```python
from build123d import *

# Parameters (mm, degrees)
BOSS_EXTRUDE1_DEPTH             = 50
BOSS_EXTRUDE2_START             = -50
BOSS_EXTRUDE2_DEPTH             = 50
F_5_0MM_CLEARANCE_DOWEL_HOLE1_D = 5
CUT_EXTRUDE1_REACH              = 67.4
SKETCH4_R                       = 5
CUT_EXTRUDE2_REACH              = 68.728
CUT_EXTRUDE3_DEPTH              = 68.194679971
TAP_DRILL_FOR_M5X0_8_TAP1_D     = 4.2
TAP_DRILL_FOR_M5X0_8_TAP1_DEPTH = 8
TAP_DRILL_FOR_M5X0_8_TAP1_TIP   = 1.2618073


with BuildPart() as part:
    # Sketch1 → Boss-Extrude1 (new body)
    with BuildSketch(Plane.XY):
        with BuildLine():
            Line((-31.734248061, 1), (-17.721808598, 1))
            ThreePointArc((-17.721808598, 1), (0, 17.75), (17.721808598, 1))
            Line((17.721808598, 1), (31.734248061, 1))
            ThreePointArc((31.734248061, 1), (0, 31.75), (-31.734248061, 1))
        make_face()
    extrude(amount=BOSS_EXTRUDE1_DEPTH)

    # Sketch9 → Boss-Extrude2 (add)
    with BuildSketch(Plane.XY.offset(50).offset(BOSS_EXTRUDE2_START)):
        with BuildLine():
            Line((31.734248061, 31.75), (0, 31.75))
            ThreePointArc((0, 31.75), (22.094258304, 22.801452805), (31.734248061, 1))
            Line((31.734248061, 1), (31.734248061, 31.75))
        make_face()
        with BuildLine():
            Line((-31.734248061, 31.75), (-31.734248061, 1))
            ThreePointArc((-31.734248061, 1), (-22.094258304, 22.801452805), (0, 31.75))
            Line((0, 31.75), (-31.734248061, 31.75))
        make_face()
    extrude(amount=BOSS_EXTRUDE2_DEPTH)

    # Ø5.0mm Clearance Dowel Hole1 (through all)
    with Locations(Plane(origin=(-24.72802833, 1, 40), x_dir=(0, 0, -1), z_dir=(0, -1, 0))):
        with Locations((0, 0), (30, 0), (0, 49.45605666), (30, 49.45605666)):
            Hole(F_5_0MM_CLEARANCE_DOWEL_HOLE1_D / 2)

    # Sketch4 → Cut-Extrude1 (cut, up to next)
    with BuildSketch(Plane(origin=(0, 4, 0), x_dir=(-1, 0, 0), z_dir=(0, -1, 0)), mode=Mode.PRIVATE) as cut_extrude1_sk1:
        with Locations(Location((24.72802833, -40, 0), (0, 0, 90))):
            Circle(SKETCH4_R)
    cut_extrude1_tool1 = extrude(cut_extrude1_sk1.sketch, amount=-CUT_EXTRUDE1_REACH, mode=Mode.PRIVATE) & part.part
    # Sketch4 → Cut-Extrude1 (cut, up to next)
    with BuildSketch(Plane(origin=(0, 4, 0), x_dir=(-1, 0, 0), z_dir=(0, -1, 0)), mode=Mode.PRIVATE) as cut_extrude1_sk2:
        with Locations(Location((24.72802833, -10, 0), (0, 0, 90))):
            Circle(SKETCH4_R)
    cut_extrude1_tool2 = extrude(cut_extrude1_sk2.sketch, amount=-CUT_EXTRUDE1_REACH, mode=Mode.PRIVATE) & part.part
    # Sketch4 → Cut-Extrude1 (cut, up to next)
    with BuildSketch(Plane(origin=(0, 4, 0), x_dir=(-1, 0, 0), z_dir=(0, -1, 0)), mode=Mode.PRIVATE) as cut_extrude1_sk3:
        with Locations(Location((-24.72802833, -10, 0), (0, 0, 90))):
            Circle(SKETCH4_R)
    cut_extrude1_tool3 = extrude(cut_extrude1_sk3.sketch, amount=-CUT_EXTRUDE1_REACH, mode=Mode.PRIVATE) & part.part
    # Sketch4 → Cut-Extrude1 (cut, up to next)
    with BuildSketch(Plane(origin=(0, 4, 0), x_dir=(-1, 0, 0), z_dir=(0, -1, 0)), mode=Mode.PRIVATE) as cut_extrude1_sk4:
        with Locations(Location((-24.72802833, -40, 0), (0, 0, 90))):
            Circle(SKETCH4_R)
    cut_extrude1_tool4 = extrude(cut_extrude1_sk4.sketch, amount=-CUT_EXTRUDE1_REACH, mode=Mode.PRIVATE) & part.part
    add(cut_extrude1_tool1.solids().sort_by_distance((-24.728028, 4, 40))[0], mode=Mode.SUBTRACT)
    add(cut_extrude1_tool2.solids().sort_by_distance((-24.728028, 4, 10))[0], mode=Mode.SUBTRACT)
    add(cut_extrude1_tool3.solids().sort_by_distance((24.728028, 4, 10))[0], mode=Mode.SUBTRACT)
    add(cut_extrude1_tool4.solids().sort_by_distance((24.728028, 4, 40))[0], mode=Mode.SUBTRACT)

    # Sketch5 → Cut-Extrude2 (cut, up to next)
    with BuildSketch(Plane(origin=(0, 1, 0), x_dir=(-1, 0, 0), z_dir=(0, -1, 0)), mode=Mode.PRIVATE) as cut_extrude2_sk1:
        with BuildLine():
            Line((-6, -35), (-6, -15))
            ThreePointArc((-6, -15), (0, -9), (6, -15))
            Line((6, -15), (6, -35))
            ThreePointArc((6, -35), (0, -41), (-6, -35))
        make_face()
    cut_extrude2_tool1 = extrude(cut_extrude2_sk1.sketch, amount=-CUT_EXTRUDE2_REACH, mode=Mode.PRIVATE) & part.part
    add(cut_extrude2_tool1.solids().sort_by_distance((0, 1, 25))[0], mode=Mode.SUBTRACT)

    # Sketch6 → Cut-Extrude3 (cut, through all)
    with BuildSketch(Plane.XY.offset(50)):
        with BuildLine():
            ThreePointArc((0, 31.75), (9.424816043, 30.318894151), (18, 26.154588508))
            Line((18, 26.154588508), (31.734248061, 26.154588508))
            Line((31.734248061, 26.154588508), (31.734248061, 31.75))
            Line((31.734248061, 31.75), (0, 31.75))
        make_face()
        with BuildLine():
            Line((18, 26.154588508), (-18, 26.154588508))
            ThreePointArc((-18, 26.154588508), (0, 31.75), (18, 26.154588508))
        make_face()
        with BuildLine():
            Line((-31.734248061, 26.154588508), (-18, 26.154588508))
            ThreePointArc((-18, 26.154588508), (-9.424816043, 30.318894151), (0, 31.75))
            Line((0, 31.75), (-31.734248061, 31.75))
            Line((-31.734248061, 31.75), (-31.734248061, 26.154588508))
        make_face()
    extrude(amount=-CUT_EXTRUDE3_DEPTH, mode=Mode.SUBTRACT)

    # Tap Drill for M5x0.8 Tap1
    with Locations(Plane(origin=(-12.5, 26.154588508, 5), x_dir=(0, 0, 1), z_dir=(0, 1, 0))):
        with Locations((0, 0), (40, 0), (40, 25), (0, 25)):
            Hole(TAP_DRILL_FOR_M5X0_8_TAP1_D / 2, depth=TAP_DRILL_FOR_M5X0_8_TAP1_DEPTH)
            with Locations((0, 0, -(TAP_DRILL_FOR_M5X0_8_TAP1_DEPTH + TAP_DRILL_FOR_M5X0_8_TAP1_TIP / 2))):  # 118° drill point
                Cone(0, TAP_DRILL_FOR_M5X0_8_TAP1_D / 2, TAP_DRILL_FOR_M5X0_8_TAP1_TIP, mode=Mode.SUBTRACT)


solid = part.part
```
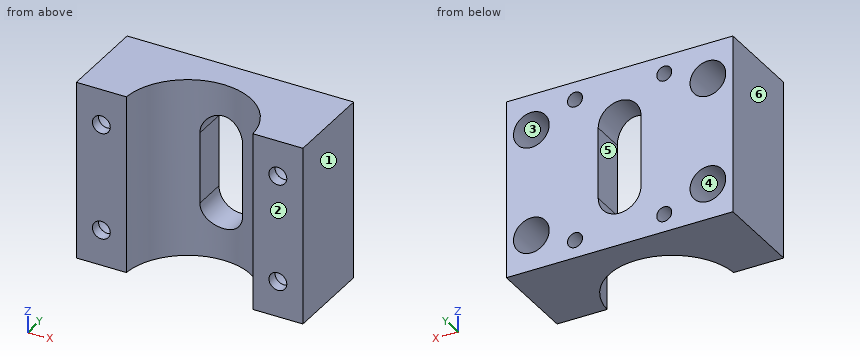
Geometry check sheet. Reference: the model listing, model coordinates, mm. Face numbers are marked on the shaded views. A direction names the side the tool comes from. Round coordinates to 2 decimals unless told otherwise and drop trailing zeros. Loops run counter-clockwise (first coordinate to the right, second up) from the corner with the lowest first, then second, coordinate; pieces in that order, holes last. Notation, with made-up numbers: (-33, -9.75) - (-2, -9.75) arc R16 ccw to (-2, 3.25) - close; hole circle Ø4 at (36.25, 44.5). An arc over 180 degrees is marked (long way). Write item = value, one per line. Start each with the question number.
1. Thickness scan on line 1 (Z direction, x = 12.5, y = 21); line 2 (X direction, y = 14.75, z = 40); line 3 (X direction, y = 2.55, z = 10). Record the ranges inside material, lowest first.
2. Section check A-A on z = 10. Enter the section's corners in (x, y), then the cut area to 3 significant figures.
3. Section check C-C on z = 36. Enter the section's corners in (x, y), then the cut area to 3 significant figures.
4. Section check B-B on y = 20.75. Give the number of separate pieces and of enclosed holes in the cut face, then the cut area to 3 significant figures.
5. Depth check by flat-ended pin: pin 1 (2.5 mm diameter, centred on x = 12.5, z = 45, fed in from -Y) (3 decimals); pin 2 (3 mm diameter, centred on x = 27, z = 9.5, fed in from +Y); pin 3 (8 mm diameter, centred on x = 1, z = 24.5, fed in from -Y); pin 4 (6.5 mm diameter, centred on x = -12.5, z = 5, fed in from -Y). Enter the tip coordinate at first touch or a pass-through.
6. Mould release check, pull along X, two halves, no side actions. Record for the marked faces 1, 2 and 3: released by +X, released by -X, zero draft, split by the parting line, or undercut.
7. Set-up check for the marked faces 4, 5 and 6: record each of +Z, -Z, +X, -X, +Y, -Y from which the full face is reachable in a straight line by a thin tool's end or side.
8. Section check D-D on x = -21. Enter the section's corners in (y, z), then the cut area to 3 significant figures.
Working result:
q1.line_1 = 0 to 2.9, 7.1 to 42.9, 47.1 to 50
q1.line_2 = -31.73 to -29.73, -19.73 to -9.87, 9.87 to 19.73, 29.73 to 31.73
q1.line_3 = -31.73 to -27.23, -22.23 to -17.57, 17.57 to 22.23, 27.23 to 31.73
q2.outline = (-31.73, 1) - (-27.23, 1) - (-27.23, 4) - (-29.73, 4) - (-29.73, 26.15) - (-31.73, 26.15) - close; (-22.23, 1) - (-17.72, 1) arc R17.75 cw to (-3.32, 17.44) - (-3.32, 26.15) - (-19.73, 26.15) - (-19.73, 4) - (-22.23, 4) - close; (3.32, 17.44) arc R17.75 cw to (17.72, 1) - (22.23, 1) - (22.23, 4) - (19.73, 4) - (19.73, 26.15) - (3.32, 26.15) - close; (27.23, 1) - (31.73, 1) - (31.73, 26.15) - (29.73, 26.15) - (29.73, 4) - (27.23, 4) - close
q2.area = 608 mm^2
q3.outline = (-31.73, 1) - (-17.72, 1) arc R17.75 cw to (-5.92, 16.74) - (-5.92, 26.15) - (-21.73, 26.15) - (-21.73, 4) - (-27.73, 4) - (-27.73, 26.15) - (-31.73, 26.15) - close; (5.92, 16.74) arc R17.75 cw to (17.72, 1) - (31.73, 1) - (31.73, 26.15) - (27.73, 26.15) - (27.73, 4) - (21.73, 4) - (21.73, 26.15) - (5.92, 26.15) - close
q3.area = 768 mm^2
q4.separate_pieces = 1
q4.enclosed_holes = 9
q4.area = 2,450 mm^2
q5.pin_1 = 11.225
q5.pin_2 = 4
q5.pin_3 = through
q5.pin_4 = 8.19
q6.face_1 = released by +X
q6.face_2 = zero draft
q6.face_3 = undercut
q7.face_4 = +Y
q7.face_5 = +Y, -Y
q7.face_6 = +Z, -Z, -X, +Y, -Y
q8.outline = (1, 0) - (26.15, 0) - (26.15, 6.67) - (4, 6.67) - (4, 13.33) - (26.15, 13.33) - (26.15, 36.67) - (4, 36.67) - (4, 43.33) - (26.15, 43.33) - (26.15, 50) - (1, 50) - close
q8.area = 962 mm^2
